Part print with two shaded views. Sizes in mm from the minimum x, y, z corner. A direction names the side the tool comes from. Coordinates: 2 decimals unless noted, no trailing zeros. Loops run counter-clockwise (first coordinate to the right, second up) from the corner with the lowest first, then second, coordinate; pieces in that order, holes last.
(1) Tool access for the marked faces 1 and 2: list every direction of +Z, -Z, +X, -X, +Y, -Y with a clear straight run to the whole face (end or side of a thin tool).
(2) Wall check: L1, parallel to Z at x = 4.5, y = 100 (3 decimals); L2, parallel to Y at x = 1.15, z = 12.7. Give the ranges that are in metal, low to high.
(3) Slice it at B-B (y = 83). Give the cut face in (x, z) (3 decimals).
(4) Slice it at A-A (x = 16.5). Give the cut face in (y, z) (3 decimals).
(5) Slice it at C-C (z = 17). Give the cut face in (x, y) (3 decimals).
(6) Two-plate mould, pull along Z, no slides. Class the marked faces 3, 4 and 5: pulls with the +Z half, pulls with the -Z half, needs draft (parallel to the pull), parting line crosses it, or undercut.
(7) Flat gauge pins, fed straight in: P1, Ø7.5, axis at y = 190.5, z = 12.7, coming from the +X side; P2, Ø4, axis at x = 4, z = 15.5, coming from the +Y side. Where does each tip first touch, or does it go through?
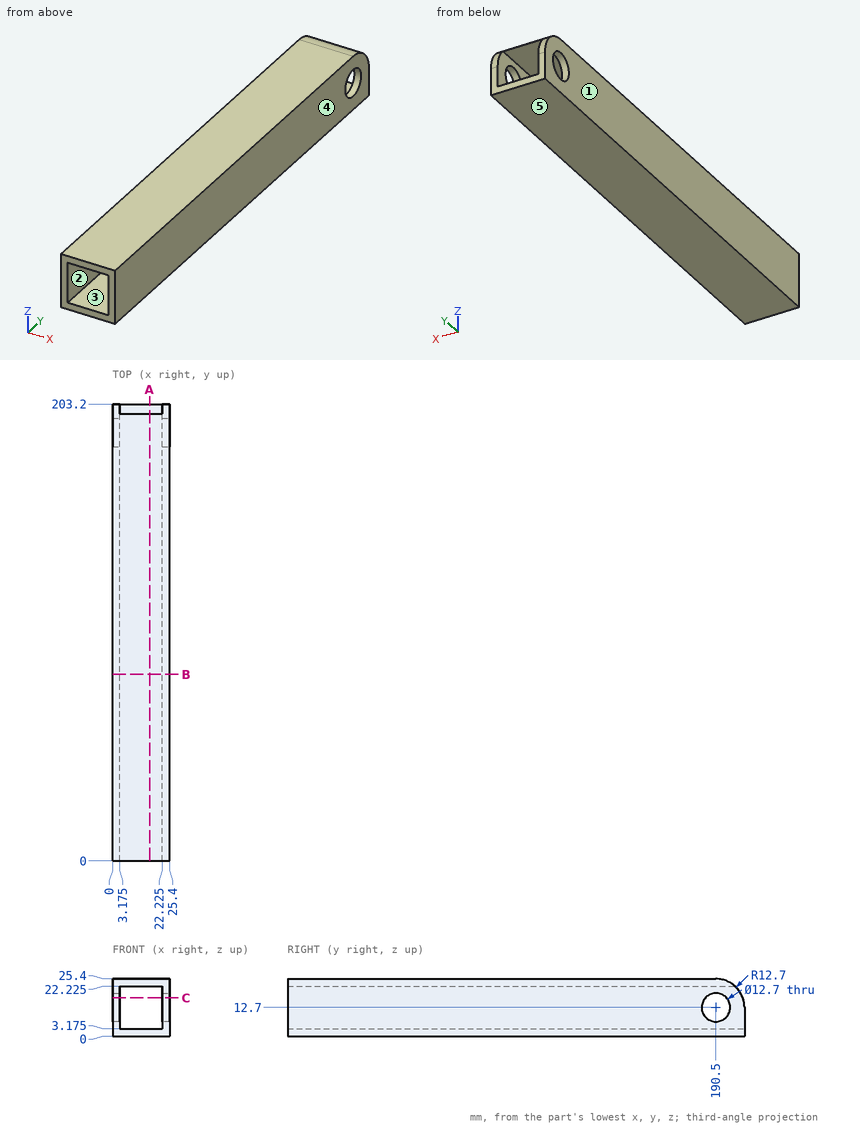
Response values:
1. face 1: +Z, -Z, -X, +Y, -Y
1. face 2: +Y, -Y
2. L1: z = 0 to 3.175, 22.225 to 25.4
2. L2: y = 0 to 184.15, 196.85 to 203.2
3. outline: (0, 0) - (25.4, 0) - (25.4, 25.4) - (0, 25.4) - close; hole (3.175, 3.175) - (22.225, 3.175) - (22.225, 22.225) - (3.175, 22.225) - close
4. outline: (0, 0) - (203.2, 0) - (203.2, 3.175) - (0, 3.175) - close; (0, 22.225) - (198.9, 22.225) arc R12.7 ccw to (190.5, 25.4) - (0, 25.4) - close
5. outline: (0, 0) - (3.175, 0) - (3.175, 185.827) - (0, 185.827) - close; (0, 195.173) - (3.175, 195.173) - (3.175, 202.45) - (0, 202.45) - close; (22.225, 0) - (25.4, 0) - (25.4, 185.827) - (22.225, 185.827) - close; (22.225, 195.173) - (25.4, 195.173) - (25.4, 202.45) - (22.225, 202.45) - close
6. face 3: undercut
6. face 4: needs draft
6. face 5: pulls with the -Z half
7. P1: passes through
7. P2: stops at y = 203.16
